Could you check a few things on this drawing? It's one solid part, dimensions in mm from its lowest x, y, z. A direction names the side the tool comes from. Give positions to 0.01 mm unless a question says otherwise; leave off trailing zeros. Loops run counter-clockwise (first coordinate to the right, second up) from the corner with the lowest first, then second, coordinate; pieces in that order, holes last. Notation, with made-up numbers: M -29.5,38 L -11.5,38 A24 ccw -11.5,69 Z; hole C -13,75 d5. An arc over 180 degrees is marked long. Return JSON: item names as keys, results as strings. Group by question number.
1. If we mould it in two halves opening along X, with no side actions, what happens to the marked faces 1, 2 and 3? For each: +X half, -X half, draft (parallel to the pull), parting line (faces both ways), or undercut.
2. If we section it at C-C (x = 15.5): Write out the boundary of the cut face in (y, z), plus the area to 3 significant figures.
3. For pin 1 (1.5 mm diameter, centred on x = 23, y = 436, fed in from +Z), with a flat end and sliding along its axis, tell me the tip position at first contact or that it passes through.
4. Please list where these lines run through material, in increasing order: line 1 (X direction, y = 193.5, z = 13); line 2 (Y direction, x = 89, z = 30.5); line 3 (Z direction, x = 40, y = 332.5).
5. For the marked faces 4 and 5, which set-ups out of +Z, -Z, +X, -X, +Y, -Y let a thin tool reach every point of the face, with its end or its side?
6. If we section it at B-B (y = 67): Write out the boundary of the cut face in (x, z).
7. If we section it at A-A (z = 27): Write out the boundary of the cut face in (x, y), plus the area to 3 significant figures.
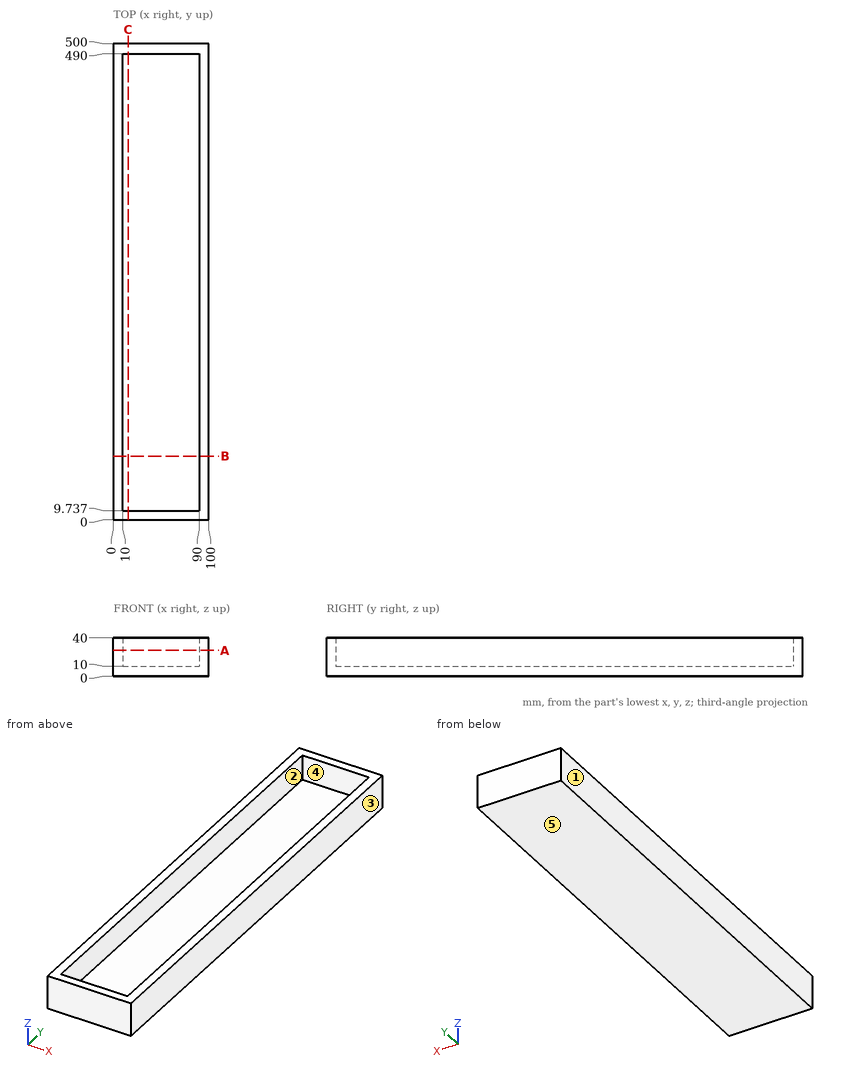
Answer:
{
 "1": {"face 1": "-X half", "face 2": "undercut", "face 3": "+X half"},
 "2": {"outline": "M 0,0 L 500,0 L 500,40 L 490,40 L 490,10 L 9.74,10 L 9.74,40 L 0,40 Z", "area": "5,590 mm²"},
 "3": {"pin 1": "stops at z = 10"},
 "4": {"line 1": "x = 0 to 10, 90 to 100", "line 2": "y = 0 to 9.74, 490 to 500", "line 3": "z = 0 to 10"},
 "5": {"face 4": "+Z", "face 5": "-Z, +X, -X, +Y, -Y"},
 "6": {"outline": "M 0,0 L 100,0 L 100,40 L 90,40 L 90,10 L 10,10 L 10,40 L 0,40 Z"},
 "7": {"outline": "M 0,0 L 100,0 L 100,500 L 0,500 Z; hole M 10,9.74 L 90,9.74 L 90,490 L 10,490 Z", "area": "11,600 mm²"}
}
